Verification items for the finished model (mm, model axes). A direction names the side the tool comes from. Round coordinates to 2 decimals unless told otherwise and drop trailing zeros. Write each loop counter-clockwise with the first axis right and the second up, starting at its lowest first coordinate (ties: lowest second). Pieces come first, ordered by that corner, then holes. Notation, with made-up numbers: M 10.5,47 L 24.5,47 A9 ccw 24.5,53 Z; hole C 4,14 d5. An arc over 180 degrees is marked long. One line per question, with ' | ' between items.
from build123d import *

# Parameters (mm, degrees)
SKETCH1_W           = 70
SKETCH1_H           = 70
SKETCH1_W_2         = 64
SKETCH1_H_2         = 64
BOSS_EXTRUDE1_DEPTH = 1000
FILLET1_R           = 5
SKETCH5_R           = 3
CUT_EXTRUDE3_DEPTH  = 70
LPATTERN1_COUNT     = 5
LPATTERN1_PITCH     = 70
LPATTERN1_COL_COUNT = 5
LPATTERN1_COL_PITCH = 70
SKETCH6_R           = 3
CUT_EXTRUDE4_DEPTH  = 70
LPATTERN2_COUNT     = 5
LPATTERN2_PITCH     = 70
LPATTERN2_COL_COUNT = 5
LPATTERN2_COL_PITCH = 70


with BuildPart() as part:
    # Sketch1 → Boss-Extrude1 (new body)
    with BuildSketch(Plane.XY):
        with Locations((35, 35)):
            Rectangle(SKETCH1_W, SKETCH1_H)
        with Locations((35, 35)):
            Rectangle(SKETCH1_W_2, SKETCH1_H_2, mode=Mode.SUBTRACT)
    extrude(amount=BOSS_EXTRUDE1_DEPTH)

    # Fillet1
    fillet1_edges = [part.edges().sort_by_distance(p)[0] for p in [
        (3, 67, 500),
        (3, 3, 500),
        (67, 3, 500),
        (67, 67, 500),
        (0, 70, 500),
        (70, 70, 500),
        (70, 0, 500),
        (0, 0, 500),
    ]]
    fillet(fillet1_edges, radius=FILLET1_R)

    # Sketch5 → Cut-Extrude3 (cut)
    with BuildSketch(Plane(origin=(0, 70, 0), x_dir=(1, 0, 0), z_dir=(0, 1, 0))):
        with Locations(Location((35, -500, 0), (0, 0, 270))):
            Circle(SKETCH5_R)
    cut_extrude3 = extrude(amount=-CUT_EXTRUDE3_DEPTH, mode=Mode.SUBTRACT)

    # LPattern1: Cut-Extrude3 ×5
    with Locations(*[(0, 0, i * LPATTERN1_PITCH) for i in range(1, LPATTERN1_COUNT)]):
        add(cut_extrude3, mode=Mode.SUBTRACT)

    # LPattern1 col: Cut-Extrude3 ×5
    with Locations(*[(0, 0, -i * LPATTERN1_COL_PITCH) for i in range(1, LPATTERN1_COL_COUNT)]):
        add(cut_extrude3, mode=Mode.SUBTRACT)

    # Sketch6 → Cut-Extrude4 (cut)
    with BuildSketch(Plane.ZY):
        with Locations(Location((500, 35, 0), (0, 0, 270))):
            Circle(SKETCH6_R)
    cut_extrude4 = extrude(amount=-CUT_EXTRUDE4_DEPTH, mode=Mode.SUBTRACT)

    # LPattern2: Cut-Extrude4 ×5
    with Locations(*[(0, 0, -i * LPATTERN2_PITCH) for i in range(1, LPATTERN2_COUNT)]):
        add(cut_extrude4, mode=Mode.SUBTRACT)

    # LPattern2 col: Cut-Extrude4 ×5
    with Locations(*[(0, 0, i * LPATTERN2_COL_PITCH) for i in range(1, LPATTERN2_COL_COUNT)]):
        add(cut_extrude4, mode=Mode.SUBTRACT)


solid = part.part
1. Thickness scan on line 1 (X direction, y = 58, z = 267.5); line 2 (Y direction, x = 5, z = 801.5). Record the ranges inside material, lowest first.
Results:
line 1: x = 0 to 3, 67 to 70 | line 2: y = 0 to 4, 66 to 70
2. Section check A-A, the plane z = 865. Record the cut outline in (x, y), then the cut area to 3 significant figures.
Results:
outline: M 0,5 A5 ccw 5,0 L 65,0 A5 ccw 70,5 L 70,65 A5 ccw 65,70 L 5,70 A5 ccw 0,65 Z; hole M 3,8 A5 ccw 8,3 L 62,3 A5 ccw 67,8 L 67,62 A5 ccw 62,67 L 8,67 A5 ccw 3,62 Z | area: 804 mm2
3. Mould release check, pull along Y, two halves, no side actions. Record for faces 3 (the face through (3, 35, 493)), 4 (the face through (35, 70, 493)), 5 (the face through (32, 1, 1000)): pulls with the +Y half, pulls with the -Y half, needs draft (parallel to the pull), parting line crosses it, or undercut.
Results:
face 3: undercut | face 4: pulls with the +Y half | face 5: needs draft
4. Tool access check on faces 1 (the face through (32, 1, 0)), 2 (the face through (35, 3, 493)). Record the directions out of +Z, -Z, +X, -X, +Y, -Y that give a thin tool (end or side, any length) a straight path to the whole face; none if there is none.
Results:
face 1: -Z, +X, -X, +Y, -Y | face 2: +Z, -Z
